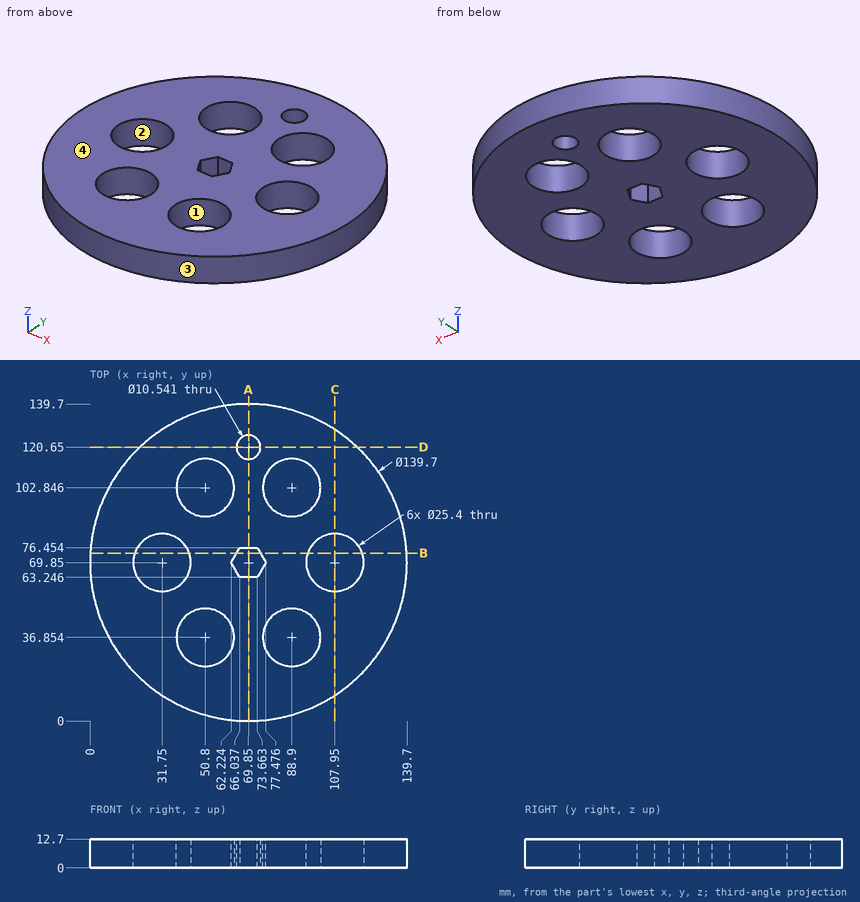
Verification items for this drawing (mm, ordinates from the low corner). Round coordinates to 2 decimals unless told otherwise and drop trailing zeros. Order: outer loops, then holes, each group sorted by start corner. A loop starts at its lowest first (then second) coordinate and runs counter-clockwise, first axis right, second up. Notation, with made-up numbers: (-23, 79.5) - (21, 79.5) arc R28 ccw to (21, 105.5) - close; hole circle Ø8 at (-35, -37). An arc over 180 degrees is marked (long way). Use CSV: the item, a comma, the result in double quotes. Start each with the question number.
1) Section check C-C, the plane x = 107.95. Record the cut outline in (y, z), plus the area to 3 significant figures.
2) Go/stop test with flat-tipped pins: P1, Ø2, axis at y = 42.5, z = 7.5, coming from the -X side; P2, Ø4, axis at x = 69, z = 4, coming from the +Y side; P3, Ø3, axis at y = 97.5, z = 9.5, coming from the +X side. Record where each tip stops, or that it passes through.
3) Section check B-B, the plane y = 74. Record the cut outline in (x, z).
4) Mould release check, pull along X, two halves, no side actions. Record for the marked faces 1, 2, 3 and 4: +X half, -X half, draft (parallel to the pull), parting line (faces both ways), or undercut.
5) Thickness scan on L1, parallel to Y at x = 69.85, z = 4.25; L2, parallel to Y at x = 88.9, z = 3.75 (1 decimal); L3, parallel to X at y = 100.5, z = 7.75 (1 decimal). Record the ranges inside material, lowest first.
6) Section check D-D, the plane y = 120.65. Record the cut outline in (x, z).
7) Section check A-A, the plane x = 69.85. Record the cut outline in (y, z).
Answers:
1,outline,"(11.31, 0) - (57.15, 0) - (57.15, 12.7) - (11.31, 12.7) - close; (82.55, 0) - (128.39, 0) - (128.39, 12.7) - (82.55, 12.7) - close"
1,area,"1,160 mm²"
2,P1,"stops at x = 5.16"
2,P2,"stops at y = 139.7"
2,P3,"stops at x = 134.62"
3,outline,"(0.12, 0) - (19.75, 0) - (19.75, 12.7) - (0.12, 12.7) - close; (43.75, 0) - (64.62, 0) - (64.62, 12.7) - (43.75, 12.7) - close; (75.08, 0) - (95.95, 0) - (95.95, 12.7) - (75.08, 12.7) - close; (119.95, 0) - (139.58, 0) - (139.58, 12.7) - (119.95, 12.7) - close"
4,face 1,"undercut"
4,face 2,"undercut"
4,face 3,"parting line"
4,face 4,"draft"
5,L1,"y = 0 to 63.25, 76.45 to 115.38, 125.92 to 139.7"
5,L2,"y = 2.6 to 24.2, 49.6 to 90.1, 115.5 to 137.1"
5,L3,"x = 7.1 to 38.3, 63.3 to 76.4, 101.4 to 132.6"
6,outline,"(21.91, 0) - (64.58, 0) - (64.58, 12.7) - (21.91, 12.7) - close; (75.12, 0) - (117.79, 0) - (117.79, 12.7) - (75.12, 12.7) - close"
7,outline,"(0, 0) - (63.25, 0) - (63.25, 12.7) - (0, 12.7) - close; (76.45, 0) - (115.38, 0) - (115.38, 12.7) - (76.45, 12.7) - close; (125.92, 0) - (139.7, 0) - (139.7, 12.7) - (125.92, 12.7) - close"
